Input: part model. Units: mm. Frame: model coordinates. A direction names the side the tool comes from. Give positions to 0.01 mm unless a question says otherwise; leave off trailing zeros. Loops run counter-clockwise (first coordinate to the right, second up) from the corner with the lowest first, then second, coordinate; pieces in that order, holes last. Notation, with made-up numbers: (25.5, 14) - (36.5, 14) arc R26 cw to (36.5, 51) - close; hole circle Ø3 at (67.25, 43.5). An arc over 180 degrees is marked (long way). Answer as a JSON object with one key per item and string values.
from build123d import *

# Parameters (mm, degrees)
SKETCH_W        = 20
SKETCH_H        = 40.5
PAD_DEPTH       = 30
SKETCH001_W     = 20
SKETCH001_H     = 53.5
PAD001_DEPTH    = 2
SKETCH002_R     = 2.15
POCKET_DEPTH    = 162.939917
PAD002_DEPTH    = 6
SKETCH004_R     = 2.5
PAD003_DEPTH    = 5
POCKET001_DEPTH = 20.001


with BuildPart() as part:
    # Sketch → Pad (new body)
    with BuildSketch(Plane.XY):
        Rectangle(SKETCH_W, SKETCH_H)
    extrude(amount=-PAD_DEPTH)

    # Sketch001 (on Face5 of Pad) → Pad001 (join)
    with BuildSketch(Plane.XY):
        Rectangle(SKETCH001_W, SKETCH001_H)
    extrude(amount=PAD001_DEPTH)

    # Sketch002 (on Face5 of Pad001) → Pocket (cut, through all)
    with BuildSketch(Plane.XY.offset(2)):
        with Locations((-5, -24.75)):
            Circle(SKETCH002_R)
        with Locations((-5, 24.75)):
            Circle(SKETCH002_R)
    pocket = extrude(amount=-POCKET_DEPTH, mode=Mode.SUBTRACT)

    # Mirrored: Pocket across Sketch002 V_Axis
    add(pocket.mirror(Plane(origin=(0, 0, 2), x_dir=(0, 0, 1), z_dir=(1, 0, 0))), mode=Mode.SUBTRACT)

    # Sketch003 (on Face4 of Mirrored) → Pad002 (join)
    with BuildSketch(Plane.XY.offset(2)):
        with BuildLine():
            ThreePointArc((10, 10.25), (0, 20.25), (-10, 10.25))
            Line((-10, -20.25), (-10, 10.25))
            Line((10, -20.25), (-10, -20.25))
            Line((10, 10.25), (10, -20.25))
        make_face()
    extrude(amount=PAD002_DEPTH)

    # Sketch004 (on Face23 of Pad002) → Pad003 (join)
    with BuildSketch(Plane.XY.offset(8)):
        with Locations((0, 10.25)):
            Circle(SKETCH004_R)
    extrude(amount=PAD003_DEPTH)

    # Sketch005 (on Face22 of Pad003) → Pocket001 (cut, through all)
    with BuildSketch(Plane.YZ.offset(10)):
        Polygon((-20.25, 2), (-9.857695, 8), (-20.25, 8), align=None)
    extrude(amount=-POCKET001_DEPTH, mode=Mode.SUBTRACT)


solid = part.part
Item 1: Mould query, pull axis Y, two halves, no side actions, for faces 1 (the face through (0.14, -15.127, 4.958)), 2 (the face through (-4.92, -22.6, 1.01)), 3 (the face through (-5.08, 22.6, 1.01)), 4 (the face through (-0.5, 7.8, 10.5)). Classes: released by +Y, released by -Y, zero draft, split by the parting line, or undercut.
Geometry check:
{"face 1": "released by -Y", "face 2": "undercut", "face 3": "undercut", "face 4": "split by the parting line"}
Item 2: Cut plane D-D (y = 9). Return loops of the section in (x, z).
Geometry check:
{"outline": "(-10, -30) - (10, -30) - (10, 8) - (2.17, 8) - (2.17, 13) - (-2.17, 13) - (-2.17, 8) - (-10, 8) - close"}
Item 3: Access query for faces 5 (the face through (0, 20.25, -15)), 6 (the face through (0, -23, 0)), 7 (the face through (0, -23, 2)), 8 (the face through (0.22, 20.248, 4.958)). Directions: +Z, -Z, +X, -X, +Y, -Y. A direction counts if a zero-diameter tool reaches every point of the face in a straight line with its end or side. Return the directions, or none.
Geometry check:
{"face 5": "-Z, +X, -X, +Y", "face 6": "-Z, +X, -X, -Y", "face 7": "+Z, +X, -X, -Y", "face 8": "+Z, +Y"}
Item 4: Cut plane C-C (z = -26). Return loops of the section in (x, y), then the cut area to 3 significant figures.
Geometry check:
{"outline": "(-10, -20.25) - (10, -20.25) - (10, 20.25) - (-10, 20.25) - close", "area": "810 mm2"}
Item 5: Cut plane B-B (x = 8). Return loops of the section in (y, z).
Geometry check:
{"outline": "(-26.75, 0) - (-20.25, 0) - (-20.25, -30) - (20.25, -30) - (20.25, 0) - (26.75, 0) - (26.75, 2) - (16.25, 2) - (16.25, 8) - (-9.86, 8) - (-20.25, 2) - (-26.75, 2) - close"}
Item 6: Cut plane A-A (y = -24.75). Return loops of the section in (x, z).
Geometry check:
{"outline": "(-10, 0) - (-7.15, 0) - (-7.15, 2) - (-10, 2) - close; (-2.85, 0) - (2.85, 0) - (2.85, 2) - (-2.85, 2) - close; (7.15, 0) - (10, 0) - (10, 2) - (7.15, 2) - close"}
Item 7: Material intervals for line 1 (X direction, y = 24.75, z = 1); line 2 (Y direction, x = 5, z = 1); line 3 (Z direction, x = -1, y = 13), sorted ascending. Write a range as [from, to].
Geometry check:
{"line 1": "x = [-10, -7.15], [-2.85, 2.85], [7.15, 10]", "line 2": "y = [-22.6, 22.6]", "line 3": "z = [-30, 8]"}
Item 8: Contact query for flat-ended pins moving along their axis: P1, Ø2, axis at x = -4, y = 24.5, coming from the -Z side; P2, Ø5, axis at x = 5, y = -24.75, coming from the +Z side; P3, Ø1, axis at x = 1, z = -19, coming from the +Y side; P4, Ø4, axis at x = -4.5, z = -10.5, coming from the -Y side. Output: stop coordinate, or through.
Geometry check:
{"P1": "passes through", "P2": "stops at z = 2", "P3": "stops at y = 20.25", "P4": "stops at y = -20.25"}
